Part model, mm, in its own coordinate system. Round coordinates to 2 decimals unless told otherwise and drop trailing zeros. Write each loop counter-clockwise with the first axis right and the second up, starting at its lowest first coordinate (ties: lowest second). Pieces come first, ordered by that corner, then holes. Notation, with made-up numbers: (42.5, -18.5) -> (60.5, -18.5) arc R12 cw to (60.5, -1.5) -> close; hole circle Ø4 at (46, 68). An arc over 180 degrees is marked (long way). Use CSV: the item, a comma, the result in double quotes. Start each with the question number.
```python
from build123d import *

# Parameters (mm, degrees)
BOSS_EXTRUDE2_DEPTH = 15
SKETCH2_R           = 18
SKETCH2_R_2         = 11
BOSS_EXTRUDE3_DEPTH = 2.5


with BuildPart() as part:
    # Sketch1 → Boss-Extrude2 (new body)
    with BuildSketch(Plane.XY):
        with BuildLine():
            ThreePointArc((28.989440912, 10.982363845), (30.493217838, 5.582442643), (31, 0))
            Line((31, 0), (40, 0))
            ThreePointArc((40, 0), (9.75236872, 38.792928535), (-35.244565217, 18.91614714))
            ThreePointArc((-35.244565217, 18.91614714), (-38.754967124, 15.524494065), (-43.582703214, 14.80394124))
            ThreePointArc((-43.582703214, 14.80394124), (-55.714436376, 11.429336197), (-61, 0))
            Line((-61, 0), (-50.5, 0))
            ThreePointArc((-50.5, 0), (-46, 4.5), (-41.5, 0))
            Line((-41.5, 0), (-31, 0))
            ThreePointArc((-31, 0), (-30.493217838, 5.582442643), (-28.989440912, 10.982363845))
            ThreePointArc((-28.989440912, 10.982363845), (-31.176914536, 18), (-24.005726539, 19.614410349))
            ThreePointArc((-24.005726539, 19.614410349), (-15.5, 26.846787517), (-4.983714373, 30.596774194))
            ThreePointArc((-4.983714373, 30.596774194), (-0.201777274, 35.995926934), (5, 31))
            ThreePointArc((5, 31), (4.995926934, 30.798222726), (4.983714373, 30.596774194))
            ThreePointArc((4.983714373, 30.596774194), (15.5, 26.846787517), (24.005726539, 19.614410349))
            ThreePointArc((24.005726539, 19.614410349), (29.17000674, 19.927488277), (31.846787517, 15.5))
            ThreePointArc((31.846787517, 15.5), (31.072498521, 12.827292288), (28.989440912, 10.982363845))
        make_face()
        with BuildLine():
            Line((40, 0), (31, 0))
            ThreePointArc((31, 0), (30.493217838, -5.582442643), (28.989440912, -10.982363845))
            ThreePointArc((28.989440912, -10.982363845), (31.072498521, -12.827292288), (31.846787517, -15.5))
            ThreePointArc((31.846787517, -15.5), (29.17000674, -19.927488277), (24.005726539, -19.614410349))
            ThreePointArc((24.005726539, -19.614410349), (15.5, -26.846787517), (4.983714373, -30.596774194))
            ThreePointArc((4.983714373, -30.596774194), (4.995926934, -30.798222726), (5, -31))
            ThreePointArc((5, -31), (-0.201777274, -35.995926934), (-4.983714373, -30.596774194))
            ThreePointArc((-4.983714373, -30.596774194), (-15.5, -26.846787517), (-24.005726539, -19.614410349))
            ThreePointArc((-24.005726539, -19.614410349), (-31.176914536, -18), (-28.989440912, -10.982363845))
            ThreePointArc((-28.989440912, -10.982363845), (-30.493217838, -5.582442643), (-31, 0))
            Line((-31, 0), (-41.5, 0))
            ThreePointArc((-41.5, 0), (-46, -4.5), (-50.5, 0))
            Line((-50.5, 0), (-61, 0))
            ThreePointArc((-61, 0), (-55.714436376, -11.429336197), (-43.582703214, -14.80394124))
            ThreePointArc((-43.582703214, -14.80394124), (-38.754967124, -15.524494065), (-35.244565217, -18.91614714))
            ThreePointArc((-35.244565217, -18.91614714), (9.75236872, -38.792928535), (40, 0))
        make_face()
        with BuildLine():
            ThreePointArc((-23, 0), (0, 23), (23, 0))
            Line((23, 0), (31, 0))
            ThreePointArc((31, 0), (30.493217838, 5.582442643), (28.989440912, 10.982363845))
            ThreePointArc((28.989440912, 10.982363845), (22.516660498, 13), (24.005726539, 19.614410349))
            ThreePointArc((24.005726539, 19.614410349), (15.5, 26.846787517), (4.983714373, 30.596774194))
            ThreePointArc((4.983714373, 30.596774194), (0, 26), (-4.983714373, 30.596774194))
            ThreePointArc((-4.983714373, 30.596774194), (-15.5, 26.846787517), (-24.005726539, 19.614410349))
            ThreePointArc((-24.005726539, 19.614410349), (-22.41929924, 17.823219222), (-21.846787517, 15.5))
            ThreePointArc((-21.846787517, 15.5), (-24.174079805, 11.274288996), (-28.989440912, 10.982363845))
            ThreePointArc((-28.989440912, 10.982363845), (-30.493217838, 5.582442643), (-31, 0))
            Line((-31, 0), (-23, 0))
        make_face()
        with BuildLine():
            Line((31, 0), (23, 0))
            ThreePointArc((23, 0), (0, -23), (-23, 0))
            Line((-23, 0), (-31, 0))
            ThreePointArc((-31, 0), (-30.493217838, -5.582442643), (-28.989440912, -10.982363845))
            ThreePointArc((-28.989440912, -10.982363845), (-24.174079805, -11.274288996), (-21.846787517, -15.5))
            ThreePointArc((-21.846787517, -15.5), (-22.41929924, -17.823219222), (-24.005726539, -19.614410349))
            ThreePointArc((-24.005726539, -19.614410349), (-15.5, -26.846787517), (-4.983714373, -30.596774194))
            ThreePointArc((-4.983714373, -30.596774194), (0, -26), (4.983714373, -30.596774194))
            ThreePointArc((4.983714373, -30.596774194), (15.5, -26.846787517), (24.005726539, -19.614410349))
            ThreePointArc((24.005726539, -19.614410349), (22.516660498, -13), (28.989440912, -10.982363845))
            ThreePointArc((28.989440912, -10.982363845), (30.493217838, -5.582442643), (31, 0))
        make_face()
    extrude(amount=-BOSS_EXTRUDE2_DEPTH)

    # Sketch2 → Boss-Extrude3 (add, symmetric)
    # profile 1 of 3: a face of its own
    with BuildSketch(Plane.XY.offset(-7.5)):
        with BuildLine():
            ThreePointArc((12.269141221, 73.170731707), (16.505219507, 67.181763642), (18, 60))
            ThreePointArc((18, 60), (6.03836873, 43.043051481), (-13.94867812, 48.623076923))
            ThreePointArc((-13.94867812, 48.623076923), (-12.352807509, 41.768456097), (-16.790075515, 36.305555556))
            ThreePointArc((-16.790075515, 36.305555556), (21.545266062, 33.701654415), (40, 0))
            ThreePointArc((40, 0), (21.545266062, -33.701654415), (-16.790075515, -36.305555556))
            ThreePointArc((-16.790075515, -36.305555556), (-12.352807509, -41.768456097), (-13.94867812, -48.623076923))
            ThreePointArc((-13.94867812, -48.623076923), (6.03836873, -43.043051481), (18, -60))
            ThreePointArc((18, -60), (16.505219507, -67.181763642), (12.269141221, -73.170731707))
            ThreePointArc((12.269141221, -73.170731707), (44.10724555, 0), (12.269141221, 73.170731707))
        make_face()
    # profile 2 of 3: a face of its own
    with BuildSketch(Plane.XY.offset(-7.5)):
        with Locations((0, 60)):
            Circle(SKETCH2_R)
        with Locations((0, 60)):
            Circle(SKETCH2_R_2, mode=Mode.SUBTRACT)
    # profile 3 of 3: a face of its own
    with BuildSketch(Plane.XY.offset(-7.5)):
        with Locations((0, -60)):
            Circle(SKETCH2_R)
        with Locations((0, -60)):
            Circle(SKETCH2_R_2, mode=Mode.SUBTRACT)
    extrude(amount=BOSS_EXTRUDE3_DEPTH, both=True)


solid = part.part
```
1. Band-saw the part on A-A (x = 0). Give the number of separate pieces and of enclosed holes in the cut face, then the cut area to 3 significant figures.
2. Pull direction X, two halves, no side cores. Call faces 1 (the cylindrical face through (-12.33, 41.87, -7.46)), 2 (the flat face through (-22, 9, 0)), 3 (the cylindrical face through (-1.432, 70.906, -7.535)): released by +X, released by -X, zero draft, split by the parting line, or undercut.
3. Band-saw the part on B-B (x = -46). List the corners of the cut face in (y, z), then the cut area to 3 significant figures.
4. Band-saw the part on D-D (y = 60). List the corners of the cut face in (x, z).
5. Drill centre lines: line 1 along X through (y, z) = (-19.5, -3); line 2 along Y through (x, z) = (-46, -7.5); line 3 along X through (y, z) = (17, -6.75). Where is each one in solid material? Low to high. Write a range as [from, to].
6. Flat gauge pins, fed straight in: pin 1 (6 mm diameter, centred on x = -29.5, z = -2.5, fed in from -Y); pin 2 (2 mm diameter, centred on y = -15, z = -3.5, fed in from +X); pin 3 (6 mm diameter, centred on x = -4, z = -8, fed in from +Y); pin 4 (20 mm diameter, centred on x = 0, y = 60, fed in from -Z). Where does each tip first touch, or does it go through?
Answers below:
1,separate pieces,"6"
1,enclosed holes,"0"
1,area,"370 mm^2"
2,face 1,"released by -X"
2,face 2,"zero draft"
2,face 3,"undercut"
3,outline,"(-15, -15) -> (-4.5, -15) -> (-4.5, 0) -> (-15, 0) -> close; (4.5, -15) -> (15, -15) -> (15, 0) -> (4.5, 0) -> close"
3,area,"315 mm^2"
4,outline,"(-18, -10) -> (-11, -10) -> (-11, -5) -> (-18, -5) -> close; (11, -10) -> (24.11, -10) -> (24.11, -5) -> (11, -5) -> close"
5,line 1,"x = [-34.92, -29.85], [-23.85, -12.2], [12.2, 23.85], [29.85, 34.92]"
5,line 2,"y = [-15, -4.5], [4.5, 15]"
5,line 3,"x = [-36.68, -31.62], [-22.08, -15.49], [15.49, 22.08], [31.62, 42.65]"
6,pin 1,"stops at y = -29.96"
6,pin 2,"stops at x = 37.47"
6,pin 3,"stops at y = 77.97"
6,pin 4,"passes through"
